For this review, take the finished solid that the model builds, in its own axes (mm). Face numbers are marked on the shaded views. A direction names the side the tool comes from. Give positions to 0.01 mm unless a question says otherwise; leave off trailing zeros. Order: outer loops, then holes, each group sorted by start corner. A loop starts at its lowest first (then second) coordinate and runs counter-clockwise, first axis right, second up. Notation, with made-up numbers: (-13, 58.25) -> (-6, 58.25) arc R12 ccw to (-6, 65.25) -> close; hole circle Ø6 at (69, -31). An arc over 180 degrees is marked (long way). Return JSON: item names as keys, results as strings. Group by question number.
1) Insertion check: P1, Ø3, axis at y = 2.5, z = 3.5, coming from the -X side; P2, Ø3, axis at y = 1.5, z = 12, coming from the +X side; P3, Ø1.5, axis at x = 3, y = 3.5, coming from the +Z side. Each pin has a flat end and moves straight along its axis. Give the tip position at first contact, or say it passes through.
2) Add section B-B (y = 2.5). Give the boundary of the cut face in (x, z), then the cut area to 3 significant figures.
3) For the marked faces 1, 2 and 3, list the 3-axis set-ups (+Z, -Z, +X, -X, +Y, -Y) from which the entire face can be reached by the end or side of a thin tool; tool diameter is ignored.
4) Add section C-C (y = 4.4). Give the boundary of the cut face in (x, z).
5) To check wall thickness, follow line 1 along X through (y, z) = (2.5, 31.4); line 2 along Z through (x, y) = (5, 1.9); line 3 along X through (y, z) = (2.5, 0.25). State the ranges of each line that lie inside material, in increasing order.
6) Add section A-A (x = 2.5). Give the boundary of the cut face in (y, z).
7) Add section D-D (x = 29.5). Give the boundary of the cut face in (y, z), then the cut area to 3 significant figures.
Autodesk Inventor part; units mm, degrees
ref_plane "YZ Plane" through (0, 0, 0) normal (1, 0, 0) x (0, 1, 0)
ref_plane "XZ Plane" through (0, 0, 0) normal (0, 1, 0) x (-1, 0, 0)
ref_plane "XY Plane" through (0, 0, 0) normal (0, 0, 1) x (1, 0, 0)
sketch "Sketch1" plane through (0, 0, 0) normal (0, 0, 1) x (1, 0, 0)
  point P0 (0, 0)
sketch "Sketch2" plane through (0, 0, 0) normal (0, 0, 1) x (1, 0, 0)
  line L0 (0, 0) -> (9.852, 0)
  line L1 (9.852, 0) -> (9.852, 5)
  line L2 (9.852, 5) -> (0, 5)
  line L3 (0, 5) -> (0, 0)
  dimension "d0" = 5
  dimension "d1" = 9.852
extrude "Plate1" add sketch "Sketch2" along normal blind 0.5
sketch "Sketch3" plane through (9.852, 5, 0.5) normal (0.8660254, 0, -0.5) x (0, 1, 0)
  line L0 (-5, 0) -> (0, 0)
  line L1 (0, 0) -> (0, 35.507)
  line L2 (0, 35.507) -> (-5, 35.507)
  line L3 (-5, 35.507) -> (-5, 0)
edge flange "Flange1" height 35.7957 angle 60 thickness 0.5 bend radius 0.5 thickness toward (0.8660254, 0, -0.5) relief tear relief width 0.5 relief depth 0.25 edges at (9.852, 2.5, 0.5) wall of the first edge with corners at (9.852, 0, 0.5) (9.852, 5, 0.5) (27.6055, 5, 31.25) (27.6055, 0, 31.25)
bend "Bend1"
corner "Corner1"
sketch "Sketch4" plane through (28.0385, 0, 31) normal (0, 0, 1) x (1, 0, 0)
  line L0 (0, 5) -> (0, 0)
  line L1 (0, 0) -> (5.7113, 0)
  line L2 (5.7113, 0) -> (5.7113, 5)
  line L3 (5.7113, 5) -> (0, 5)
edge flange "Flange2" height 6 angle 60 thickness 0.5 bend radius 0.5 thickness toward (0, 0, 1) relief tear relief width 0.5 relief depth 0.25 edges at (28.0385, 2.5, 31) wall of the first edge with corners at (28.0385, 5, 31) (28.0385, 0, 31) (33.7499, 0, 31) (33.7499, 5, 31)
bend "Bend2"
corner "Corner2"
sketch "Sketch5" plane through (0, 0, 0) normal (0, 0, -1) x (-1, 0, 0)
  line L0 (-9.5633, 5) -> (-9.5633, 0)
  line L1 (0, 5) -> (0, 0)
  line L2 (0, 2.5) -> (-9.5633, 2.5) construction
  point P0 (-2.5, 2.5)
  dimension "d23" = 2.5
hole "Hole1" at (2.5, 2.5, 0) direction (0, 0, 1) diameter 2.5 depth 0.5 tip angle 118
sketch "Sketch6" plane through (33.7499, 0, 31) normal (0, 0, -1) x (-1, 0, 0)
  line L0 (5.4226, 0) -> (5.4226, 5)
  line L1 (0, 5) -> (0, 0)
  line L2 (0, 2.5) -> (5.4226, 2.5) construction
  point P0 (33.7498, 0)
  point P1 (2.5, 2.5)
  dimension "d31" = 2.5
hole "Hole2" at (31.2499, 2.5, 31) direction (0, 0, 1) diameter 2.5 depth 0.5 tip angle 118
fillet "Corner Round1" radius 2 4 edges at (0, 5, 0.25) (0, 0, 0.25) (33.7499, 0, 31.25) (33.7499, 5, 31.25)
equation "\"d29\" = Thickness"
equation "\"d37\" = Thickness"
equation "\"d3\" = BendReliefWidth"
equation "\"d4\" = BendReliefDepth"
equation "\"d5\" = MinimumRemnant"
equation "\"d6\" = BendRadius"
equation "\"d9\" = BendRadius"
equation "\"d10\" = CornerReliefSize"
equation "\"d11\" = GapSize"
equation "\"d12\" = JacobiRadiusSize"
equation "\"d13\" = BendReliefWidth"
equation "\"d14\" = BendReliefDepth"
equation "\"d15\" = MinimumRemnant"
equation "\"d16\" = BendRadius"
equation "\"d19\" = BendRadius"
equation "\"d20\" = CornerReliefSize"
equation "\"d21\" = GapSize"
equation "\"d22\" = JacobiRadiusSize"
equation "\"BendRadius\" = Thickness"
equation "\"BendReliefWidth\" = Thickness"
equation "\"BendReliefDepth\" = 0.5 * Thickness"
equation "\"CornerReliefSize\" = 4 * Thickness"
equation "\"MinimumRemnant\" = 2 * Thickness"
equation "\"TransitionRadius\" = BendRadius"
equation "\"JacobiRadiusSize\" = BendRadius"
equation "\"GapSize\" = Thickness"
equation "\"d2\" = BendRadius"
properties part number "core_earth_new" material "Copper, Cast"
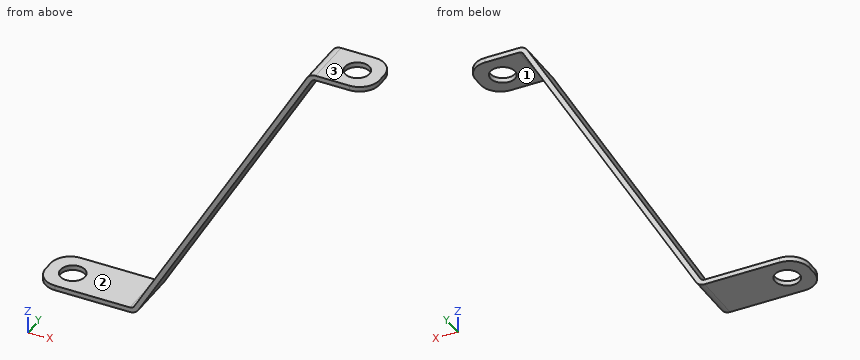
Evaluation:
{
 "1": {"P1": "x = 10.72", "P2": "x = 17.93", "P3": "z = 0.5"},
 "2": {"outline": "(0, 0) -> (1.25, 0) -> (1.25, 0.5) -> (0, 0.5) -> close; (3.75, 0) -> (9.56, 0) arc R1 ccw to (10.43, 0.5) -> (27.89, 30.75) arc R0.5 cw to (28.33, 31) -> (30, 31) -> (30, 31.5) -> (28.33, 31.5) arc R1 ccw to (27.46, 31) -> (10, 0.75) arc R0.5 cw to (9.56, 0.5) -> (3.75, 0.5) -> close; (32.5, 31) -> (33.75, 31) -> (33.75, 31.5) -> (32.5, 31.5) -> close", "area": "23.2 mm^2"},
 "3": {"face 1": "-Z, +X, +Y, -Y", "face 2": "+Z, -X, +Y, -Y", "face 3": "+Z, +X, -X, +Y, -Y"},
 "4": {"outline": "(0.57, 0) -> (9.56, 0) arc R1 ccw to (10.43, 0.5) -> (27.89, 30.75) arc R0.5 cw to (28.33, 31) -> (33.18, 31) -> (33.18, 31.5) -> (28.33, 31.5) arc R1 ccw to (27.46, 31) -> (10, 0.75) arc R0.5 cw to (9.56, 0.5) -> (0.57, 0.5) -> close"},
 "5": {"line 1": "27.89 to 30, 32.5 to 33.75", "line 2": "0 to 0.5", "line 3": "0 to 1.25, 3.75 to 10.22"},
 "6": {"outline": "(0, 0) -> (1.25, 0) -> (1.25, 0.5) -> (0, 0.5) -> close; (3.75, 0) -> (5, 0) -> (5, 0.5) -> (3.75, 0.5) -> close"},
 "7": {"outline": "(0, 31) -> (5, 31) -> (5, 31.5) -> (0, 31.5) -> close", "area": "2.50 mm^2"}
}
